Source: three-view drawing plus pictorial views. Frame: mm from the lowest corner of the part. A direction names the side the tool comes from. Give positions to 0.01 mm unless a question says otherwise; leave off trailing zeros. Loops run counter-clockwise (first coordinate to the right, second up) from the corner with the lowest first, then second, coordinate; pieces in that order, holes last. Notation, with made-up numbers: M 28,41.25 L 72,41.25 A34 ccw 72,78.25 Z; hole C 69.25,31.5 d2. An arc over 180 degrees is marked long. Write item = value, one per line.
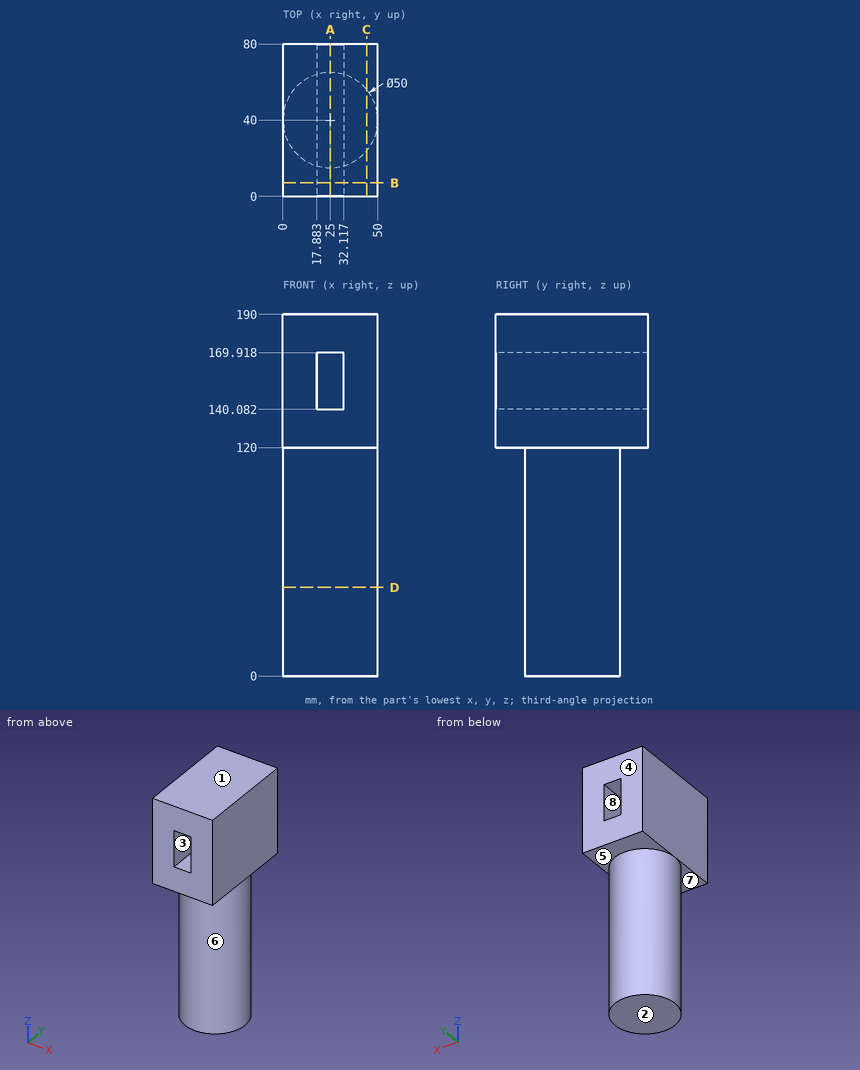
1. Pull-direction query (Z, two-part tool) for the marked faces 1, 2 and 3; classes: +Z half, -Z half, draft (parallel to the pull), parting line (faces both ways), or undercut.
Derived:
face_1 = +Z half
face_2 = -Z half
face_3 = undercut
2. Cut plane C-C, the plane x = 44. Return the cut outline in (y, z).
Derived:
outline = M 0,120 L 23.75,120 L 23.75,0 L 56.25,0 L 56.25,120 L 80,120 L 80,190 L 0,190 Z
3. Cut plane B-B, the plane y = 7. Return the cut outline in (x, z).
Derived:
outline = M 0,120 L 50,120 L 50,190 L 0,190 Z; hole M 17.88,140.08 L 32.12,140.08 L 32.12,169.92 L 17.88,169.92 Z
4. Cut plane D-D, the plane z = 46.5. Return the cut outline in (x, y), then the cut area to 3 significant figures.
Derived:
outline = C 25,40 d50
area = 1,960 mm²
5. Reachability of the marked faces 4, 5, 6, 7 and 8 from +Z, -Z, +X, -X, +Y, -Y: full face, straight path, thin tool, end or side. Return the list, or none.
Derived:
face_4 = +Z, -Z, +X, -X, +Y
face_5 = -Z, +Y
face_6 = -Z
face_7 = -Z, -Y
face_8 = +Y, -Y
6. Cut plane A-A, the plane x = 25. Return the cut outline in (y, z).
Derived:
outline = M 0,120 L 15,120 L 15,0 L 65,0 L 65,120 L 80,120 L 80,140.08 L 0,140.08 Z; M 0,169.92 L 80,169.92 L 80,190 L 0,190 Z
7. First-contact query: pin 1 Ø2 at (x, z) = (42.5, 59) entering from -Y; pin 2 Ø6 at (y, z) = (23.5, 105.5) entering from -X; pin 3 Ø8 at (x, z) = (6, 35) entering from -Y. Flat tips, straight axial feed; report the tip coordinate or a pass-through.
Derived:
pin_1 = 21.22
pin_2 = 3.96
pin_3 = 20
8. Material intervals for probe 1 along Z at (x, y) = (29.5, 37.5); probe 2 along X at (y, z) = (16.5, 146); probe 3 along Z at (x, y) = (4, 74.5), sorted ascending. Write a range as from..to.
Derived:
probe_1 = 0..140.08, 169.92..190
probe_2 = 0..17.88, 32.12..50
probe_3 = 120..190
